```python
from build123d import *

# Parameters (mm, degrees)
SKETCH_1_R      = 29.5
SKETCH_1_R_2    = 5.05
SKETCH_1_R_3    = 4
SKETCH_1_W      = 8.1
SKETCH_1_H      = 2.1
EXTRUDE_1_DEPTH = 2


with BuildPart() as part:
    # 草图1 → 凸台-拉伸1 (new body)
    with BuildSketch(Plane.XY):
        with Locations((0, 4)):
            Circle(SKETCH_1_R)
        with Locations((0, 4)):
            Circle(SKETCH_1_R_2, mode=Mode.SUBTRACT)
        with Locations((0, -20.5)):
            Circle(SKETCH_1_R_3, mode=Mode.SUBTRACT)
        with Locations((-15, 4)):
            Rectangle(SKETCH_1_W, SKETCH_1_H, mode=Mode.SUBTRACT)
        with Locations((-15, 0)):
            Rectangle(SKETCH_1_W, SKETCH_1_H, mode=Mode.SUBTRACT)
        with Locations((15, 4)):
            Rectangle(SKETCH_1_W, SKETCH_1_H, mode=Mode.SUBTRACT)
        with Locations((15, 0)):
            Rectangle(SKETCH_1_W, SKETCH_1_H, mode=Mode.SUBTRACT)
    extrude(amount=EXTRUDE_1_DEPTH)


solid = part.part
```
Design review of the part built by this model. Coordinates are the model's own, in mm. A direction names the side the tool comes from. Coordinates: 2 decimals unless noted, no trailing zeros. Order: outer loops, then holes, each group sorted by start corner. A loop starts at its lowest first (then second) coordinate and runs counter-clockwise, first axis right, second up. Notation, with made-up numbers: (50.25, 34) -> (64.25, 34) arc R16 cw to (64.25, 53) -> close; hole circle Ø5 at (77, 39). An arc over 180 degrees is marked (long way). One line per item, written item: value. Start each with the question number.
Q1. Take a section at D-D, the plane y = -19.5. State the section outline as (x, z) points, then the cut area to 3 significant figures.
Q2. Mouldability with a two-part tool opening along X and no side actions: class faces 3 (the flat face through (6, 4, 0)), 4 (the cylindrical face through (28.14, 12.86, 0.99)), 5 (the flat face through (15, 2.95, 1)) as pulls with the +X half, pulls with the -X half, needs draft (parallel to the pull), parting line crosses it, or undercut.
Q3. Take a section at C-C, the plane z = 0.6. State the section outline as (x, y) points, then the cut area to 3 significant figures.
Q4. Insertion check: pin 1 Ø0.6 at (y, z) = (0, 0.5) entering from +X; pin 2 Ø0.6 at (y, z) = (3.5, 1.5) entering from +X; pin 3 Ø6.5 at (x, y) = (0, -20.5) entering from +Z; pin 4 Ø0.6 at (x, z) = (16, 1) entering from +Y. Each pin has a flat end and moves straight along its axis. Give the tip position at first contact, or say it passes through.
Q5. Tool access review of faces 1 (the flat face through (-15, 1.05, 1)), 2 (the flat face through (6, 4, 2)): name each direction out of +Z, -Z, +X, -X, +Y, -Y from which nothing blocks a thin tool from reaching the whole face with its end or side.
Q6. For probe 1 along Y at (x, z) = (0, 1.25); probe 2 along Y at (x, z) = (-18.5, 0.85); probe 3 along X at (y, z) = (5, 0.15), list the stretches that pass through material, from the lowest coordinate up.
Q7. Take a section at B-B, the plane y = 4. State the section outline as (x, z) points.
Q8. Take a section at A-A, the plane x = 0. State the section outline as (y, z) points, then the cut area to 3 significant figures.
Values follow:
1. outline: (-17.83, 0) -> (-3.87, 0) -> (-3.87, 2) -> (-17.83, 2) -> close; (3.87, 0) -> (17.83, 0) -> (17.83, 2) -> (3.87, 2) -> close
1. area: 55.8 mm2
2. face 3: needs draft
2. face 4: parting line crosses it
2. face 5: undercut
3. outline: circle Ø59 at (0, 4); hole (-19.05, -1.05) -> (-10.95, -1.05) -> (-10.95, 1.05) -> (-19.05, 1.05) -> close; hole (-19.05, 2.95) -> (-10.95, 2.95) -> (-10.95, 5.05) -> (-19.05, 5.05) -> close; hole circle Ø10.1 at (0, 4); hole circle Ø8 at (0, -20.5); hole (10.95, -1.05) -> (19.05, -1.05) -> (19.05, 1.05) -> (10.95, 1.05) -> close; hole (10.95, 2.95) -> (19.05, 2.95) -> (19.05, 5.05) -> (10.95, 5.05) -> close
3. area: 2,540 mm2
4. pin 1: stops at x = 29.27
4. pin 2: stops at x = 29.5
4. pin 3: passes through
4. pin 4: stops at y = 28.98
5. face 1: +Z, -Z
5. face 2: +Z, +X, -X, +Y, -Y
6. probe 1: y = -25.5 to -24.5, -16.5 to -1.05, 9.05 to 33.5
6. probe 2: y = -18.98 to -1.05, 1.05 to 2.95, 5.05 to 26.98
6. probe 3: x = -29.48 to -19.05, -10.95 to -4.95, 4.95 to 10.95, 19.05 to 29.48
7. outline: (-29.5, 0) -> (-19.05, 0) -> (-19.05, 2) -> (-29.5, 2) -> close; (-10.95, 0) -> (-5.05, 0) -> (-5.05, 2) -> (-10.95, 2) -> close; (5.05, 0) -> (10.95, 0) -> (10.95, 2) -> (5.05, 2) -> close; (19.05, 0) -> (29.5, 0) -> (29.5, 2) -> (19.05, 2) -> close
8. outline: (-25.5, 0) -> (-24.5, 0) -> (-24.5, 2) -> (-25.5, 2) -> close; (-16.5, 0) -> (-1.05, 0) -> (-1.05, 2) -> (-16.5, 2) -> close; (9.05, 0) -> (33.5, 0) -> (33.5, 2) -> (9.05, 2) -> close
8. area: 81.8 mm2
